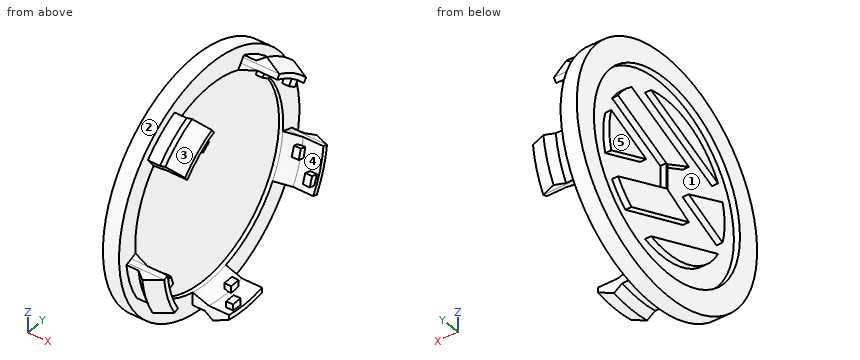
from build123d import *

# Parameters (mm, degrees)
CUT_EXTRUDE_1_DEPTH      = 9
SKETCH_4_W               = 1.7
SKETCH_4_H               = 2.5
EXTRUDE_1_DEPTH          = 2
PATTERN_CIRCULAR_1_COUNT = 5
SKETCH_5_R               = 24.3
CUT_EXTRUDE_2_DEPTH      = 1.5


with BuildPart() as part:
    # Эскиз1 → Повернуть1 (revolve)
    with BuildSketch(Plane.XY, mode=Mode.PRIVATE) as revolve_1_sk:
        Polygon((0, 30), (4, 30), (4, 26), (3, 26), (3, 0), (0, 0), align=None)
    revolve(revolve_1_sk.sketch.rotate(Axis((0, 0, 0), (-1, 0, 0)), 90), axis=Axis((0, 0, 0), (-1, 0, 0)))

    # Эскиз2 → Повернуть2 (revolve)
    with BuildSketch(Plane.XY, mode=Mode.PRIVATE) as revolve_2_sk:
        Polygon((4, 24.594119063), (8, 26.05), (13, 26.05), (13, 27.25), (9, 29.25), (7, 27.75), (3, 27.75), (3, 24.594119063), align=None)
    revolve(revolve_2_sk.sketch.rotate(Axis((0, 0, 0), (1, 0, 0)), 90), axis=Axis((0, 0, 0), (1, 0, 0)))

    # Эскиз3 → Вырез-Вытянуть1 (cut)
    with BuildSketch(Plane(origin=(13, 0, 0), x_dir=(0, 0, -1), z_dir=(1, 0, 0))):
        with BuildLine():
            ThreePointArc((13.478222015, -23.68332813), (22.045713097, -16.017148125), (26.689183202, -5.5))
            Line((26.689183202, -5.5), (25.462766935, -5.5))
            ThreePointArc((25.462766935, -5.5), (21.074892703, -15.311805822), (13.099238546, -22.516936948))
            Line((13.099238546, -22.516936948), (13.478222015, -23.68332813))
        make_face()
        with BuildLine():
            ThreePointArc((13.099238546, -22.516936948), (21.074892703, -15.311805822), (25.462766935, -5.5))
            Line((25.462766935, -5.5), (23.971247203, -5.5))
            ThreePointArc((23.971247203, -5.5), (19.897060284, -14.456060478), (12.638333602, -21.098417387))
            Line((12.638333602, -21.098417387), (13.099238546, -22.516936948))
        make_face()
        with BuildLine():
            ThreePointArc((-18.359183889, -20.137101751), (-8.420713097, -25.916290069), (3.016600336, -27.082515068))
            Line((3.016600336, -27.082515068), (2.637616867, -25.916123886))
            ThreePointArc((2.637616867, -25.916123886), (-8.049892703, -24.775022249), (-17.366992287, -19.416232356))
            Line((-17.366992287, -19.416232356), (-18.359183889, -20.137101751))
        make_face()
        with BuildLine():
            ThreePointArc((-17.366992287, -19.416232356), (-8.049892703, -24.775022249), (2.637616867, -25.916123886))
            Line((2.637616867, -25.916123886), (2.176711923, -24.497604325))
            ThreePointArc((2.176711923, -24.497604325), (-7.600000752, -23.390397197), (-16.160327476, -18.539539054))
            Line((-16.160327476, -18.539539054), (-17.366992287, -19.416232356))
        make_face()
        with BuildLine():
            Line((-23.832630062, 10.517045418), (-24.824821664, 11.237914813))
            ThreePointArc((-24.824821664, 11.237914813), (-27.25, 0), (-24.824821664, -11.237914813))
            Line((-24.824821664, -11.237914813), (-23.832630062, -10.517045418))
            ThreePointArc((-23.832630062, -10.517045418), (-26.05, 0), (-23.832630062, 10.517045418))
        make_face()
        with BuildLine():
            Line((-22.625965251, 9.640352116), (-23.832630062, 10.517045418))
            ThreePointArc((-23.832630062, 10.517045418), (-26.05, 0), (-23.832630062, -10.517045418))
            Line((-23.832630062, -10.517045418), (-22.625965251, -9.640352116))
            ThreePointArc((-22.625965251, -9.640352116), (-24.594119063, 0), (-22.625965251, 9.640352116))
        make_face()
        with BuildLine():
            Line((2.637616867, 25.916123886), (3.016600336, 27.082515068))
            ThreePointArc((3.016600336, 27.082515068), (-8.420713097, 25.916290069), (-18.359183889, 20.137101751))
            Line((-18.359183889, 20.137101751), (-17.366992287, 19.416232356))
            ThreePointArc((-17.366992287, 19.416232356), (-8.049892703, 24.775022249), (2.637616867, 25.916123886))
        make_face()
        with BuildLine():
            Line((2.176711923, 24.497604325), (2.637616867, 25.916123886))
            ThreePointArc((2.637616867, 25.916123886), (-8.049892703, 24.775022249), (-17.366992287, 19.416232356))
            Line((-17.366992287, 19.416232356), (-16.160327476, 18.539539054))
            ThreePointArc((-16.160327476, 18.539539054), (-7.600000752, 23.390397197), (2.176711923, 24.497604325))
        make_face()
        with BuildLine():
            Line((25.462766935, 5.5), (26.689183202, 5.5))
            ThreePointArc((26.689183202, 5.5), (22.045713097, 16.017148125), (13.478222015, 23.68332813))
            Line((13.478222015, 23.68332813), (13.099238546, 22.516936948))
            ThreePointArc((13.099238546, 22.516936948), (21.074892703, 15.311805822), (25.462766935, 5.5))
        make_face()
        with BuildLine():
            Line((23.971247203, 5.5), (25.462766935, 5.5))
            ThreePointArc((25.462766935, 5.5), (21.074892703, 15.311805822), (13.099238546, 22.516936948))
            Line((13.099238546, 22.516936948), (12.638333602, 21.098417387))
            ThreePointArc((12.638333602, 21.098417387), (19.897060284, 14.456060478), (23.971247203, 5.5))
        make_face()
        with BuildLine():
            Line((3.016600336, 27.082515068), (4.573471173, 31.874070813))
            ThreePointArc((4.573471173, 31.874070813), (-9.950505703, 30.624507588), (-22.435124657, 23.09844606))
            Line((-22.435124657, 23.09844606), (-18.359183889, 20.137101751))
            ThreePointArc((-18.359183889, 20.137101751), (-8.420713097, 25.916290069), (3.016600336, 27.082515068))
        make_face()
        with BuildLine():
            Line((-24.824821664, 11.237914813), (-28.900762432, 14.199259122))
            ThreePointArc((-28.900762432, 14.199259122), (-32.200512865, 0), (-28.900762432, -14.199259122))
            Line((-28.900762432, -14.199259122), (-24.824821664, -11.237914813))
            ThreePointArc((-24.824821664, -11.237914813), (-27.25, 0), (-24.824821664, 11.237914813))
        make_face()
        with BuildLine():
            ThreePointArc((-22.435124657, -23.09844606), (-9.950505703, -30.624507588), (4.573471173, -31.874070813))
            Line((4.573471173, -31.874070813), (3.016600336, -27.082515068))
            ThreePointArc((3.016600336, -27.082515068), (-8.420713097, -25.916290069), (-18.359183889, -20.137101751))
            Line((-18.359183889, -20.137101751), (-22.435124657, -23.09844606))
        make_face()
        with BuildLine():
            ThreePointArc((15.035092852, -28.474883875), (26.050762135, -18.926986578), (31.727323063, -5.5))
            Line((31.727323063, -5.5), (26.689183202, -5.5))
            ThreePointArc((26.689183202, -5.5), (22.045713097, -16.017148125), (13.478222015, -23.68332813))
            Line((13.478222015, -23.68332813), (15.035092852, -28.474883875))
        make_face()
        with BuildLine():
            Line((26.689183202, 5.5), (31.727323063, 5.5))
            ThreePointArc((31.727323063, 5.5), (26.050762135, 18.926986578), (15.035092852, 28.474883875))
            Line((15.035092852, 28.474883875), (13.478222015, 23.68332813))
            ThreePointArc((13.478222015, 23.68332813), (22.045713097, 16.017148125), (26.689183202, 5.5))
        make_face()
    extrude(amount=-CUT_EXTRUDE_1_DEPTH, mode=Mode.SUBTRACT)

    # Эскиз4 → Бобышка-Вытянуть1 (add)
    with BuildSketch(Plane.XY.offset(-24.3)):
        with Locations((11.65, -2.25)):
            Rectangle(SKETCH_4_W, SKETCH_4_H)
        with Locations((7.85, 2.25)):
            Rectangle(SKETCH_4_W, SKETCH_4_H)
    extrude_1 = extrude(amount=-EXTRUDE_1_DEPTH)

    # Круговой массив1: Бобышка-Вытянуть1 ×5 about axis
    pattern_circular_1_axis = Axis((0, 0, 0), (1, 0, 0))
    for i in range(1, PATTERN_CIRCULAR_1_COUNT):
        add(extrude_1.rotate(pattern_circular_1_axis, i * 360 / PATTERN_CIRCULAR_1_COUNT))

    # Эскиз5 → Вырез-Вытянуть2 (cut)
    with BuildSketch(Plane(origin=(0, 0, 0), x_dir=(0, 0, -1), z_dir=(1, 0, 0))):
        with Locations(Location((0, 0, 0), (0, 0, 180))):
            Circle(SKETCH_5_R)
        with BuildLine():
            Line((-5.087573742, 18.513686651), (0, 6.870909772))
            Line((0, 6.870909772), (5.087573742, 18.513686651))
            ThreePointArc((5.087573742, 18.513686651), (0, 19.2), (-5.087573742, 18.513686651))
        make_face(mode=Mode.SUBTRACT)
        with BuildLine():
            Line((-10.213287696, 16.25819038), (-3.196299518, 0.2))
            Line((-3.196299518, 0.2), (3.196299518, 0.2))
            Line((3.196299518, 0.2), (10.213287696, 16.25819038))
            ThreePointArc((10.213287696, 16.25819038), (12.879492014, 14.239335851), (15.154936685, 11.788464449))
            Line((15.154936685, 11.788464449), (6.970698587, -7.322816425))
            Line((6.970698587, -7.322816425), (3.180185716, -0.2))
            Line((3.180185716, -0.2), (-3.180185716, -0.2))
            Line((-3.180185716, -0.2), (-6.970698587, -7.322816425))
            Line((-6.970698587, -7.322816425), (-15.154936685, 11.788464449))
            ThreePointArc((-15.154936685, 11.788464449), (-12.879492014, 14.239335851), (-10.213287696, 16.25819038))
        make_face(mode=Mode.SUBTRACT)
        with BuildLine():
            Line((-8.901263668, -17.011981223), (-18.454870493, 5.296957155))
            ThreePointArc((-18.454870493, 5.296957155), (-17.649694103, -7.558326406), (-8.901263668, -17.011981223))
        make_face(mode=Mode.SUBTRACT)
        with BuildLine():
            Line((0, -7.230363982), (-5.083762601, -18.514733534))
            ThreePointArc((-5.083762601, -18.514733534), (0, -19.2), (5.083762601, -18.514733534))
            Line((5.083762601, -18.514733534), (0, -7.230363982))
        make_face(mode=Mode.SUBTRACT)
        with BuildLine():
            Line((8.901263668, -17.011981223), (18.454870493, 5.296957155))
            ThreePointArc((18.454870493, 5.296957155), (17.649694103, -7.558326406), (8.901263668, -17.011981223))
        make_face(mode=Mode.SUBTRACT)
    extrude(amount=CUT_EXTRUDE_2_DEPTH, mode=Mode.SUBTRACT)


solid = part.part
Can you work these out from the model? Positions are in its coordinate system, mm. Face numbers are marked on the shaded views. A direction names the side the tool comes from. Round coordinates to 2 decimals unless told otherwise and drop trailing zeros. Order: outer loops, then holes, each group sorted by start corner. A loop starts at its lowest first (then second) coordinate and runs counter-clockwise, first axis right, second up. Notation, with made-up numbers: (-9, 75.5) -> (12, 75.5) arc R10 ccw to (12, 94.5) -> close; hole circle Ø3 at (-9.75, 66). An arc over 180 degrees is marked (long way). Write each question's results on one line, items separated by ' | '. Start each with the question number.
Item 1: Please list where these lines run through material, in increasing order: L1, parallel to Z at x = 1.25, y = -2.5; L2, parallel to X at y = 3, z = 25; L3, parallel to X at y = -19.5, z = 9.5.
Item 2: Which directions (+Z, -Z, +X, -X, +Y, -Y) give clear straight access to the entire face, cutting with the end or side of a thin tool? Please do the marked faces 4 and 5.
Item 3: Thinking about a two-plate mould opening in Y: for the marked faces 1, 2 and 3, which applies, +Y half, -Y half, draft (parallel to the pull), parting line (faces both ways), or undercut?
Item 4: Will these pins go through, and if not, where does the flat tip stop? pin 1 (1 mm diameter, centred on y = -7.5, z = 2.5, fed in from -X); pin 2 (3 mm diameter, centred on x = 10, z = -13.5, fed in from +Y); pin 3 (2.5 mm diameter, centred on y = -16, z = 18.5, fed in from +X).
Item 5: If we section it at A-A, the plane z = 11: Write out the boundary of the cut face in (x, y).
Results:
1) L1: z = -29.9 to -24.17, -19.04 to -15.12, -9.04 to -4.4, 4.4 to 9.04, 15.12 to 19.04, 24.17 to 29.9 | L2: x = 0 to 4 | L3: x = 1.5 to 3
2) face 4: none | face 5: +Z, -Z, -X, +Y, -Y
3) face 1: undercut | face 2: parting line | face 3: -Y half
4) pin 1: stops at x = 1.5 | pin 2: stops at y = 26.5 | pin 3: stops at x = 8.7
5) outline: (0, -27.91) -> (4, -27.91) -> (4, -22) -> (3, -22) -> (3, 22) -> (4, 22) -> (4, 27.91) -> (0, 27.91) -> (0, 21.67) -> (1.5, 21.67) -> (1.5, 15.74) -> (0, 15.74) -> (0, 2.09) -> (1.5, 2.09) -> (1.5, -12.11) -> (0, -12.11) -> (0, -15.74) -> (1.5, -15.74) -> (1.5, -21.67) -> (0, -21.67) -> close
